from build123d import *

# Parameters (mm, degrees)
PAD_DEPTH            = 10
SKETCH_W             = 20
SKETCH_H             = 8
PAD001_DEPTH         = 5
POCKET_DEPTH         = 2.5
SKETCH003_R          = 1.6
POCKET001_DEPTH      = 20.001
SKETCH004_R          = 1.6
POCKET002_DEPTH      = 10.001
POCKET002_DEPTH_BACK = -10.001


with BuildPart() as part:
    # Sketch001 → Pad (new body)
    with BuildSketch(Plane.XY):
        Polygon((-1.9, 0), (-3.5, 1.6), (-1.6, 1.6), (0, 0), (1.6, 1.6), (3.5, 1.6), (1.9, 0), (1.9, -20), (-1.9, -20), align=None)
    extrude(amount=PAD_DEPTH)

    # Sketch → Pad001 (join)
    with BuildSketch(Plane.XZ):
        with Locations((0, 4)):
            Rectangle(SKETCH_W, SKETCH_H)
    extrude(amount=PAD001_DEPTH)

    # Sketch002 → Pocket (cut)
    with BuildSketch(Plane.XZ):
        Polygon((-3.125, 2.340118), (-3.125, 5.659882), (-6, 7.319764), (-8.875, 5.659882), (-8.875, 2.340118), (-6, 0.680236), align=None)
        Polygon((3.125, 2.340118), (6, 0.680236), (8.875, 2.340118), (8.875, 5.659882), (6, 7.319764), (3.125, 5.659882), align=None)
    extrude(amount=POCKET_DEPTH, mode=Mode.SUBTRACT)

    # Sketch003 → Pocket001 (cut, through all)
    with BuildSketch(Plane.XZ):
        with Locations((-6, 4)):
            Circle(SKETCH003_R)
        with Locations((6, 4)):
            Circle(SKETCH003_R)
    extrude(amount=POCKET001_DEPTH, mode=Mode.SUBTRACT)

    # Sketch004 → Pocket002 (cut, two sides)
    with BuildSketch(Plane.YZ) as pocket002_sk:
        with Locations((-15, 5)):
            Circle(SKETCH004_R)
    extrude(amount=-POCKET002_DEPTH, mode=Mode.SUBTRACT)
    extrude(pocket002_sk.sketch, amount=-POCKET002_DEPTH_BACK, mode=Mode.SUBTRACT)


solid = part.part
Verification items for the finished model (mm, model axes). A direction names the side the tool comes from. Coordinates: 2 decimals unless noted, no trailing zeros. Write each loop counter-clockwise with the first axis right and the second up, starting at its lowest first coordinate (ties: lowest second). Pieces come first, ordered by that corner, then holes. Notation, with made-up numbers: (23, 31.25) - (57, 31.25) arc R29 ccw to (57, 53.25) - close; hole circle Ø5 at (32, 41). An arc over 180 degrees is marked (long way). Answer as a JSON object with one key per item and string values.
(1) Cross-section at A-A on y = -15. Record the cut outline in (x, z), plus the area to 3 significant figures.
Report:
{"outline": "(-1.9, 0) - (1.9, 0) - (1.9, 3.4) - (-1.9, 3.4) - close; (-1.9, 6.6) - (1.9, 6.6) - (1.9, 10) - (-1.9, 10) - close", "area": "25.8 mm^2"}
(2) Cross-section at C-C on z = 6.25. Record the cut outline in (x, y).
Report:
{"outline": "(-10, -5) - (-1.9, -5) - (-1.9, -14) - (1.9, -14) - (1.9, -5) - (10, -5) - (10, 0) - (7.85, 0) - (7.85, -2.5) - (4.15, -2.5) - (4.15, 0) - (1.9, 0) - (3.5, 1.6) - (1.6, 1.6) - (0, 0) - (-1.6, 1.6) - (-3.5, 1.6) - (-1.9, 0) - (-4.15, 0) - (-4.15, -2.5) - (-7.85, -2.5) - (-7.85, 0) - (-10, 0) - close; (-1.9, -20) - (1.9, -20) - (1.9, -16) - (-1.9, -16) - close"}
(3) Cross-section at D-D on z = 5. Give the number of separate pieces and of enclosed holes in the cut face, plus the area to 3 significant figures.
Report:
{"separate pieces": "4", "enclosed holes": "0", "area": "110 mm^2"}
(4) Tool access check on faces 1 (the flat face through (-6, -2, 8)), 2 (the flat face through (6, -2, 8)), 3 (the flat face through (-2.7, 0.8, 4.9)), 4 (the flat face through (-8.875, -1, 4)), 5 (the flat face through (-3.125, -1, 4)). Record the directions out of +Z, -Z, +X, -X, +Y, -Y that give a thin tool (end or side, any length) a straight path to the whole face; none if there is none.
Report:
{"face 1": "+Z, -X, -Y", "face 2": "+Z, +X, -Y", "face 3": "+Z, -Z, -X", "face 4": "+Y", "face 5": "none"}
(5) Thickness scan on line 1 along X through (y, z) = (-4.1, 4); line 2 along X through (y, z) = (-1.25, 2.75) (3 decimals); line 3 along Z through (x, y) = (6, -3.9). Record the ranges inside material, lowest first.
Report:
{"line 1": "-10 to -7.6, -4.4 to 4.4, 7.6 to 10", "line 2": "-10 to -8.875, -3.125 to 3.125, 8.875 to 10", "line 3": "0 to 2.4, 5.6 to 8"}
(6) Mould release check, pull along Y, two halves, no side actions. Record for faces 6 (the flat face through (1, 1, 5)), 7 (the cylindrical face through (0.03, -16.6, 5.07)), 8 (the flat face through (-10, -2, 4)), 9 (the flat face through (6, -5, 6)): pulls with the +Y half, pulls with the -Y half, needs draft (parallel to the pull), parting line crosses it, or undercut.
Report:
{"face 6": "pulls with the +Y half", "face 7": "undercut", "face 8": "needs draft", "face 9": "pulls with the -Y half"}
(7) Gauge pin test, flat ends, axial feed: pin 1 Ø5 at (y, z) = (-15, 5) entering from -X; pin 2 Ø3 at (x, z) = (-6, 4) entering from +Y; pin 3 Ø5.5 at (x, y) = (-5, -2.5) entering from +Z; pin 4 Ø4 at (x, z) = (7, 4) entering from +Y. Record the tip position at first contact, or that the pin passes through.
Report:
{"pin 1": "x = -1.9", "pin 2": "through", "pin 3": "z = 8", "pin 4": "y = 0"}
(8) Cross-section at B-B on x = -0.25. Record the cut outline in (y, z), plus the area to 3 significant figures.
Report:
{"outline": "(-20, 0) - (0.25, 0) - (0.25, 10) - (-20, 10) - close; hole circle Ø3.2 at (-15, 5)", "area": "194 mm^2"}
